from build123d import *

# Parameters (mm, degrees)
SKETCH1_R                = 42.5
SKETCH1_R_2              = 5
BOSS_EXTRUDE1_DEPTH      = 5
SKETCH2_R                = 1.2
SKETCH2_R_2              = 1.225
SKETCH2_R_3              = 5.05
SKETCH2_R_4              = 1.015
CUT_EXTRUDE1_DEPTH       = 10
SKETCH5_R                = 5
SKETCH5_R_2              = 1.015
BOSS_EXTRUDE2_DEPTH      = 6
SKETCH9_R                = 2.357259082
BOSS_EXTRUDE4_DEPTH      = 1
FILLET1_R                = 1
SKETCH10_R               = 1.5
CUT_EXTRUDE3_DEPTH       = 2.2
CUT_EXTRUDE3_DEPTH_BACK  = 16
CUT_EXTRUDE6_DEPTH       = 0.5
CUT_EXTRUDE7_DEPTH       = 10
CUT_EXTRUDE8_DEPTH       = 10
CUT_EXTRUDE8_DEPTH_BACK  = 10
CUT_EXTRUDE9_DEPTH       = 10
CUT_EXTRUDE9_DEPTH_BACK  = 10
SKETCH17_R               = 5.5
CUT_EXTRUDE10_DEPTH      = 10
CUT_EXTRUDE10_DEPTH_BACK = 10
SKETCH18_R               = 2.25
CUT_EXTRUDE11_DEPTH      = 2.2


with BuildPart() as part:
    # Sketch1 → Boss-Extrude1 (new body)
    with BuildSketch(Plane(origin=(0, 0, 0), x_dir=(1, 0, 0), z_dir=(0, 1, 0))):
        Circle(SKETCH1_R)
        with Locations((-7.573934673, -17.06033615)):
            Circle(SKETCH1_R_2, mode=Mode.SUBTRACT)
    extrude(amount=BOSS_EXTRUDE1_DEPTH)

    # Sketch2 → Cut-Extrude1 (cut)
    with BuildSketch(Plane(origin=(0, 5, 0), x_dir=(1, 0, 0), z_dir=(0, 1, 0))):
        with Locations((26.030814012, 7.899159566)):
            Circle(SKETCH2_R)
        with Locations((17.087578103, 21.16635714)):
            Circle(SKETCH2_R)
        with Locations((13.062426036, 8.805202225)):
            Circle(SKETCH2_R_2)
        with Locations((21.559196058, 14.532758353)):
            Circle(SKETCH2_R_3)
        with Locations((8.320757608, 18.248434254)):
            Circle(SKETCH2_R_4)
    extrude(amount=-CUT_EXTRUDE1_DEPTH, mode=Mode.SUBTRACT)

    # Sketch5 → Boss-Extrude2 (add)
    with BuildSketch(Plane(origin=(0, 5, 0), x_dir=(1, 0, 0), z_dir=(0, 1, 0))):
        with Locations((-7.55311225, 14.331451264)):
            Circle(SKETCH5_R)
        with Locations((-7.55311225, 14.331451264)):
            Circle(SKETCH5_R_2, mode=Mode.SUBTRACT)
    extrude(amount=BOSS_EXTRUDE2_DEPTH)

    # Sketch9 → Boss-Extrude4 (add)
    with BuildSketch(Plane.XZ):
        with Locations((8.320757608, -18.248434254)):
            Circle(SKETCH9_R)
    extrude(amount=-BOSS_EXTRUDE4_DEPTH)

    # Fillet1
    fillet1_edges = [part.edges().sort_by_distance(p)[0] for p in [
        (-42.5, 5, 0),
    ]]
    fillet(fillet1_edges, radius=FILLET1_R)

    # Sketch10 → Cut-Extrude3 (cut, two sides)
    with BuildSketch(Plane(origin=(0, 5, 0), x_dir=(1, 0, 0), z_dir=(0, 1, 0))) as cut_extrude3_sk:
        with Locations((0, 37.8)):
            Circle(SKETCH10_R)
        with Locations((-32.735760263, -18.9)):
            Circle(SKETCH10_R)
        with Locations((32.735760263, -18.9)):
            Circle(SKETCH10_R)
    extrude(amount=CUT_EXTRUDE3_DEPTH, mode=Mode.SUBTRACT)
    extrude(cut_extrude3_sk.sketch, amount=-CUT_EXTRUDE3_DEPTH_BACK, mode=Mode.SUBTRACT)

    # Sketch12 → Cut-Extrude6 (cut)
    with BuildSketch(Plane.XZ):
        with BuildLine():
            Line((-21.313834783, 24.76213107), (-34.538834783, 1.855759139))
            ThreePointArc((-34.538834783, 1.855759139), (-35.038336896, -1.938336086), (-32.708707764, -4.974367879))
            Line((-32.708707764, -4.974367879), (-14.089161583, -15.724367879))
            ThreePointArc((-14.089161583, -15.724367879), (-10.295066357, -16.223869992), (-7.259034564, -13.894240861))
            Line((-7.259034564, -13.894240861), (5.965965436, 9.01213107))
            ThreePointArc((5.965965436, 9.01213107), (0.201065327, 30.527031179), (-21.313834783, 24.76213107))
        make_face()
    extrude(amount=-CUT_EXTRUDE6_DEPTH, mode=Mode.SUBTRACT)

    # Sketch13 → Cut-Extrude7 (cut)
    with BuildSketch(Plane(origin=(0, 5, 0), x_dir=(1, 0, 0), z_dir=(0, 1, 0))):
        with BuildLine():
            Line((32.816836472, -6.07169605), (21.984996749, -21.138640776))
            ThreePointArc((21.984996749, -21.138640776), (16.391033491, -22.978825985), (12.925236211, -18.21784334))
            Line((12.925236211, -18.21784334), (12.931687147, -3.407234286))
            ThreePointArc((12.931687147, -3.407234286), (14.35531099, 0.084802692), (17.813324255, 1.589186743))
            Line((17.813324255, 1.589186743), (28.638713042, 1.845522414))
            ThreePointArc((28.638713042, 1.845522414), (33.179093412, -0.819461796), (32.816836472, -6.07169605))
        make_face()
    extrude(amount=-CUT_EXTRUDE7_DEPTH, mode=Mode.SUBTRACT)

    # Sketch15 → Cut-Extrude8 (cut, two sides)
    with BuildSketch(Plane.XZ.offset(-0.5)) as cut_extrude8_sk:
        with BuildLine():
            Line((-4.454061063, -15.186961023), (-14.190064184, -29.028285448))
            ThreePointArc((-14.190064184, -29.028285448), (-14.263329759, -31.217660805), (-12.286203391, -32.160901823))
            Line((-12.286203391, -32.160901823), (11.926297184, -28.886712635))
            ThreePointArc((11.926297184, -28.886712635), (14.476623444, -26.492368994), (13.043930349, -23.301062679))
            Line((13.043930349, -23.301062679), (-1.808225202, -14.611372289))
            ThreePointArc((-1.808225202, -14.611372289), (-3.243361659, -14.383326468), (-4.454061063, -15.186961023))
        make_face()
    extrude(amount=CUT_EXTRUDE8_DEPTH, mode=Mode.SUBTRACT)
    extrude(cut_extrude8_sk.sketch, amount=-CUT_EXTRUDE8_DEPTH_BACK, mode=Mode.SUBTRACT)

    # Sketch16 → Cut-Extrude9 (cut, two sides)
    with BuildSketch(Plane.XZ.offset(-0.5)) as cut_extrude9_sk:
        with BuildLine():
            Line((-12.984156175, 14.705600426), (-13.719701132, 11.95882482))
            ThreePointArc((-13.719701132, 11.95882482), (-13.693758532, 7.802544191), (-11.54963643, 4.241914739))
            Line((-11.54963643, 4.241914739), (-10.842839117, 3.568938111))
            ThreePointArc((-10.842839117, 3.568938111), (-9.907482144, -2.457917187), (-15.493944375, -4.905225341))
            Line((-15.493944375, -4.905225341), (-19.004093622, -4.034917019))
            ThreePointArc((-19.004093622, -4.034917019), (-20.457115896, -3.417911536), (-21.645362284, -2.3786618))
            Line((-21.645362284, -2.3786618), (-25.653320737, 2.441392154))
            ThreePointArc((-25.653320737, 2.441392154), (-26.807383132, 5.519886283), (-25.80025353, 8.649531003))
            Line((-25.80025353, 8.649531003), (-19.012059198, 17.647148968))
            ThreePointArc((-19.012059198, 17.647148968), (-14.786139745, 18.659973084), (-12.984156175, 14.705600426))
        make_face()
    extrude(amount=CUT_EXTRUDE9_DEPTH, mode=Mode.SUBTRACT)
    extrude(cut_extrude9_sk.sketch, amount=-CUT_EXTRUDE9_DEPTH_BACK, mode=Mode.SUBTRACT)

    # Sketch17 → Cut-Extrude10 (cut, two sides)
    with BuildSketch(Plane.XZ.offset(-0.5)) as cut_extrude10_sk:
        Circle(SKETCH17_R)
    extrude(amount=CUT_EXTRUDE10_DEPTH, mode=Mode.SUBTRACT)
    extrude(cut_extrude10_sk.sketch, amount=-CUT_EXTRUDE10_DEPTH_BACK, mode=Mode.SUBTRACT)

    # Sketch18 → Cut-Extrude11 (cut)
    with BuildSketch(Plane(origin=(0, 5, 0), x_dir=(1, 0, 0), z_dir=(0, 1, 0))):
        with Locations((17.087578103, 21.16635714)):
            Circle(SKETCH18_R)
        with Locations((26.030814012, 7.899159566)):
            Circle(SKETCH18_R)
    extrude(amount=-CUT_EXTRUDE11_DEPTH, mode=Mode.SUBTRACT)


solid = part.part
Source: CAD feature listing. Evaluate the final solid. Frame: model axes, mm. A direction names the side the tool comes from. Give positions to 0.01 mm unless a question says otherwise; leave off trailing zeros. Write each loop counter-clockwise with the first axis right and the second up, starting at its lowest first coordinate (ties: lowest second). Pieces come first, ordered by that corner, then holes. Notation, with made-up numbers: M 13,12 L 28,12 A37 cw 28,49 Z; hole C 61.25,-2.5 d5. An arc over 180 degrees is marked long. Return JSON: item names as keys, results as strings. Group by question number.
1) Cut plane B-B, the plane x = 0. Output: boundary loops of the cut face in (y, z), plus the area to 3 significant figures.
2) Cut plane A-A, the plane z = 0. Output: boundary loops of the cut face in (x, y), plus the area to 3 significant figures.
3) Pin query (flat end, axial travel): P1, Ø5.5, axis at x = -5.5, z = -17, coming from the -Y side; P2, Ø2, axis at x = 7, y = 5.5, coming from the -Z side; P3, Ø2, axis at x = -20, z = -3.5, coming from the -Y side; P4, Ø1.6, axis at x = 9, z = -18.5, coming from the +Y side. Return the tip coordinate at first contact, or that it passes through.
4) Material intervals for line 1 along Z through (x, y) = (-9, 4.75); line 2 along Z through (x, y) = (0, 2.8); line 3 along X through (y, z) = (3.5, -1), sorted ascending. Write a range as [from, to].
5) Set-up query: faces 1 (the face through (18, 2.8, -20)), 2 (the face through (-10.35, 0.25, -16.24)), 3 (the face through (-0.349, 2.535, -30.547)). Return all of +Z, -Z, +X, -X, +Y, -Y with unobstructed straight access to the full face (end or side cutting, diameter ignored); none if empty.
6) Pull-direction query (Z, two-part tool) for faces 4 (the face through (-14.28, 2.54, -31.19)), 5 (the face through (9, 0, -1)), 6 (the face through (-17.224, 2.718, -4.476)); classes: pulls with the +Z half, pulls with the -Z half, needs draft (parallel to the pull), parting line crosses it, or undercut.
7) Cut plane C-C, the plane y = 9.25. Output: boundary loops of the cut face in (x, z) (3 decimals), plus the area to 3 significant figures.
Recorded:
{
 "1": {"outline": "M 0,-42.5 L 4,-42.5 A1 ccw 5,-41.5 L 5,-39.3 L 0,-39.3 Z; M 0,-36.3 L 5,-36.3 L 5,-30.5 L 0,-30.5 Z; M 0,-15.67 L 5,-15.67 L 5,-5.5 L 0,-5.5 Z; M 0,30.64 L 0.5,30.64 L 0.5,5.5 L 5,5.5 L 5,41.5 A1 ccw 4,42.5 L 0,42.5 Z", "area": "268 mm²"},
 "2": {"outline": "M -42.5,0 L -35.17,0 L -35.17,0.5 L -23.62,0.5 L -23.62,5 L -41.5,5 A1 ccw -42.5,4 Z; M -9.29,0.5 L -5.5,0.5 L -5.5,5 L -9.29,5 Z; M 5.5,0 L 14.27,0 L 14.27,5 L 5.5,5 Z; M 32.64,0 L 42.5,0 L 42.5,4 A1 ccw 41.5,5 L 32.64,5 Z", "area": "198 mm²"},
 "3": {"P1": "stops at y = 0", "P2": "stops at z = -41.81", "P3": "stops at y = 0.5", "P4": "stops at y = 5"},
 "4": {"line 1": "z = [-41.19, -31.72], [-21.65, 12.27], [21.85, 41.19]", "line 2": "z = [-42.5, -39.3], [-36.3, -30.5], [-15.67, -5.5], [5.5, 42.5]", "line 3": "x = [-42.49, -22.79], [-9.38, -5.41], [5.41, 15.57], [31.54, 42.49]"},
 "5": {"face 1": "+Y", "face 2": "-Y", "face 3": "+Y, -Y"},
 "6": {"face 4": "undercut", "face 5": "needs draft", "face 6": "undercut"},
 "7": {"outline": "M -7.367,-19.328 L -4.454,-15.187 A2 cw -2.553,-14.355 A5 ccw long Z; hole C -7.553,-14.331 d2.03", "area": "65.6 mm²"}
}
